from build123d import *

# Parameters (mm, degrees)
F0_R     = 75
F0_R_2   = 30
F1_DEPTH = 5
F3_D     = 5
F5_DEPTH = 5
F7_DEPTH = 5


# Not quite as in the source:
# - a pattern or mirror of a feature is missing from the dataset's text; its kind, count and spacing are read off the source's solid


with BuildPart() as f1:
    # F0 (on Top) → F1 (new body)
    with BuildSketch(Plane.XY):
        with Locations((-0.4658745937, 0.1248266798)):
            Circle(F0_R)
        Circle(F0_R_2, mode=Mode.SUBTRACT)
    extrude(amount=F1_DEPTH)

    # F3 (through all)
    with Locations(Plane.XY.offset(5)):
        with Locations((0, 35), (33.2869780703, 10.8155948031), (20.5724838302, -28.3155948031), (-20.5724838302, -28.3155948031), (-33.2869780703, 10.8155948031)):
            Hole(F3_D / 2)

    # F4 (on face) → F5 (cut, through all)
    with BuildSketch(Plane.XY.offset(5)):
        with BuildLine():
            ThreePointArc((2.5, -35), (0, -32.5), (-2.5, -35))
            Line((-2.5, -35), (-2.5, -65))
            ThreePointArc((-2.5, -65), (0, -67.5), (2.5, -65))
            Line((2.5, -65), (2.5, -35))
        make_face()
    f5 = extrude(amount=-F5_DEPTH, mode=Mode.SUBTRACT)

    # F5_copies: F5 across plane
    add(f5.mirror(Plane.ZX), mode=Mode.SUBTRACT)

    # F6 (on face) → F7 (cut, through all)
    with BuildSketch(Plane.XY.offset(5)):
        with BuildLine():
            ThreePointArc((-60, 3), (-63, 0), (-60, -3))
            Line((-60, -3), (-35, -3))
            ThreePointArc((-35, -3), (-32, 0), (-35, 3))
            Line((-35, 3), (-60, 3))
        make_face()
    extrude(amount=-F7_DEPTH, mode=Mode.SUBTRACT)


solid = f1.part
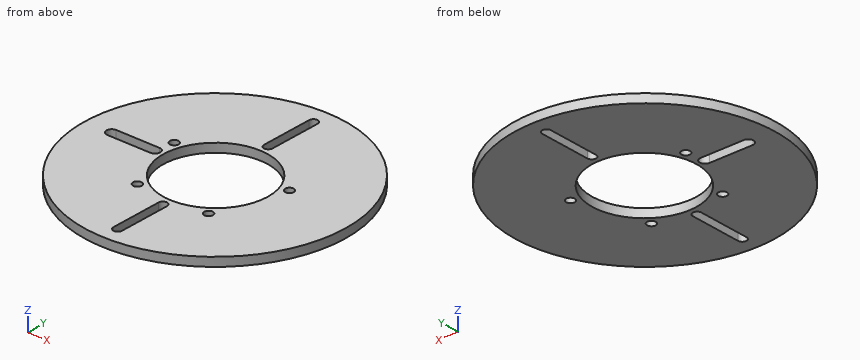
Work out the finished part from the listing and answer in its coordinate system (mm). Give positions to 0.01 mm unless a question says otherwise; leave off trailing zeros. Order: outer loops, then holes, each group sorted by start corner. A loop starts at its lowest first (then second) coordinate and runs counter-clockwise, first axis right, second up. Notation, with made-up numbers: M 45,-39 L 63,-39 A20 ccw 63,-32 Z; hole C 37.5,79 d4. An arc over 180 degrees is marked long. Return JSON: item names as keys, results as strings.
Q1. Find the intervals of material crossed by line 1 along X through (y, z) = (10, 3.6); line 2 along Y through (x, z) = (-19, 2.1); line 3 along X through (y, z) = (9, 4.35), in increasing order. Write a range as [from, to].
Answer below:
{"line 1": "x = [-74.81, -35.65], [-30.92, -28.28], [28.28, 30.92], [35.65, 73.88]", "line 2": "y = [-72.55, -30.26], [-26.37, -23.22], [23.22, 72.8]", "line 3": "x = [-74.94, -35.01], [-31.57, -28.62], [28.62, 31.57], [35.01, 74.01]"}
Q2. Find section C-C, the plane z = 1.45. State how many separate pieces and enclosed holes the cut face has, and give its area (3 significant figures).
Answer below:
{"separate pieces": "1", "enclosed holes": "8", "area": "14,200 mm^2"}
Q3. Find section B-B, the plane y = 46. Write down the section's boundary in (x, z).
Answer below:
{"outline": "M -59.8,0 L -2.5,0 L -2.5,5 L -59.8,5 Z; M 2.5,0 L 58.87,0 L 58.87,5 L 2.5,5 Z"}
Q4. Find section D-D, the plane x = -50. Write down the section's boundary in (y, z).
Answer below:
{"outline": "M -56.19,0 L -3,0 L -3,5 L -56.19,5 Z; M 3,0 L 56.44,0 L 56.44,5 L 3,5 Z"}
Q5. Each of these flat-tipped pins is pushed along its axis until it touches: pin 1 (1.5 mm diameter, centred on x = -51.5, z = 3.5, fed in from +Y); pin 2 (2.5 mm diameter, centred on x = -48, z = 3.5, fed in from -Y); pin 3 (2.5 mm diameter, centred on y = -49, z = 1.5, fed in from -X). Where does it stop, or does it pass through?
Answer below:
{"pin 1": "stops at y = 55.77", "pin 2": "stops at y = -58.89", "pin 3": "stops at x = -58.2"}
Q6. Find section A-A, the plane x = 0. Write down the section's boundary in (y, z).
Answer below:
{"outline": "M -74.87,0 L -67.5,0 L -67.5,5 L -74.87,5 Z; M -32.5,0 L -30,0 L -30,5 L -32.5,5 Z; M 30,0 L 32.5,0 L 32.5,5 L 30,5 Z; M 67.5,0 L 75.12,0 L 75.12,5 L 67.5,5 Z"}
